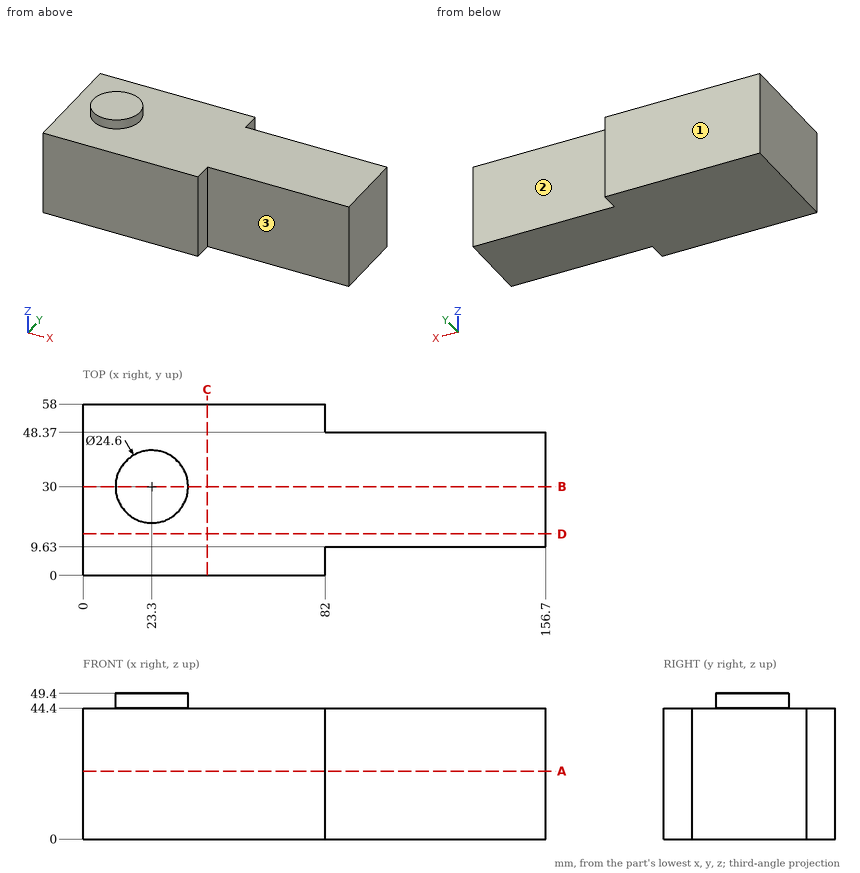
Study the drawing (mm; zero at the part's minimum x, y, z) and answer. A direction names the side the tool comes from. Coordinates: 2 decimals unless noted, no trailing zeros. Write each loop counter-clockwise with the first axis right and the second up, starting at its lowest first coordinate (ties: lowest second). Pieces come first, ordered by that corner, then holes. Notation, with made-up numbers: M 11,-30.5 L 20,-30.5 A3 ccw 20,-25.5 Z; hole C 82,12.5 d1. An arc over 180 degrees is marked long. Use a Markdown table: item, result. Add a question column.
1. Section A-A (z = 23) is taken. Give the vertices of the cut face in (x, y).
2. Section C-C (x = 42) is taken. Give the vertices of the cut face in (y, z).
3. Straight lines are drawn through the part: line 1 along Y through (x, z) = (123, 37); line 2 along Z through (x, y) = (16, 46.5); line 3 along X through (y, z) = (53.5, 27). For each, find the intervals that lie inside material, in ascending order. Write a range as [from, to].
4. Section D-D (y = 14) is taken. Give the vertices of the cut face in (x, z), plus the area to 3 significant figures.
5. Given P1, Ø1.5, axis at x = 105.5, z = 6, coming from the +Y side; P2, Ø8, axis at x = 109, z = 36.5, coming from the -Y side; P3, Ø3, axis at x = 102, y = 15, coming from the +Z side, each flat-ended and moving along its own axis, determine where each tip first touches the part or whether it passes through.
6. Section B-B (y = 30) is taken. Give the vertices of the cut face in (x, z), plus the area to 3 significant figures.
7. Which of the six approach directions +Z, -Z, +X, -X, +Y, -Y give full straight-line access (tool end or side, diameter ignored) to the marked faces 1, 2 and 3?
Data:
| question | item | result |
|---|---|---|
| 1 | outline | M 0,0 L 82,0 L 82,9.63 L 156.7,9.63 L 156.7,48.37 L 82,48.37 L 82,58 L 0,58 Z |
| 2 | outline | M 0,0 L 58,0 L 58,44.4 L 0,44.4 Z |
| 3 | line 1 | y = [9.63, 48.37] |
| 3 | line 2 | z = [0, 44.4] |
| 3 | line 3 | x = [0, 82] |
| 4 | outline | M 0,0 L 156.7,0 L 156.7,44.4 L 0,44.4 Z |
| 4 | area | 6,960 mm2 |
| 5 | P1 | stops at y = 48.37 |
| 5 | P2 | stops at y = 9.63 |
| 5 | P3 | stops at z = 44.4 |
| 6 | outline | M 0,0 L 156.7,0 L 156.7,44.4 L 35.6,44.4 L 35.6,49.4 L 11,49.4 L 11,44.4 L 0,44.4 Z |
| 6 | area | 7,080 mm2 |
| 7 | face 1 | +Z, -Z, +X, -X, +Y |
| 7 | face 2 | +Z, -Z, +X, +Y |
| 7 | face 3 | +Z, -Z, +X, -Y |
